```python
from build123d import *

# Parameters (mm, degrees)
SKETCH_1_R          = 1.45
EXTRUDE_1_DEPTH     = 3
SKETCH_3_R          = 1.95
CUT_EXTRUDE_2_DEPTH = 77.216796049
FILLET_1_R          = 5
SKETCH_4_R          = 10
CUT_EXTRUDE_3_DEPTH = 77.216796049
SKETCH_5_R          = 2.213245743
CUT_EXTRUDE_4_DEPTH = 77.216796049
FILLET_2_R          = 10
FILLET_3_R          = 3
FILLET_4_R          = 8


with BuildPart() as part:
    # 草图1 → 凸台-拉伸1 (new body)
    with BuildSketch(Plane.XY):
        with BuildLine():
            Line((-30, 31), (30, 31))
            Line((30, 31), (30, -40))
            ThreePointArc((30, -40), (0, -70), (-30, -40))
            Line((-30, -40), (-30, 31))
        make_face()
        with Locations((-20, 26)):
            Circle(SKETCH_1_R, mode=Mode.SUBTRACT)
        with Locations((-20, 16)):
            Circle(SKETCH_1_R, mode=Mode.SUBTRACT)
        with Locations((-20, 6)):
            Circle(SKETCH_1_R, mode=Mode.SUBTRACT)
        with Locations((-8, 26)):
            Circle(SKETCH_1_R, mode=Mode.SUBTRACT)
        with Locations((-8, 16)):
            Circle(SKETCH_1_R, mode=Mode.SUBTRACT)
        with Locations((-8, 6)):
            Circle(SKETCH_1_R, mode=Mode.SUBTRACT)
        with Locations(Location((8, 6, 0), (0, 0, 180))):
            Circle(SKETCH_1_R, mode=Mode.SUBTRACT)
        with Locations(Location((8, 16, 0), (0, 0, 180))):
            Circle(SKETCH_1_R, mode=Mode.SUBTRACT)
        with Locations(Location((8, 26, 0), (0, 0, 180))):
            Circle(SKETCH_1_R, mode=Mode.SUBTRACT)
        with Locations(Location((20, 6, 0), (0, 0, 180))):
            Circle(SKETCH_1_R, mode=Mode.SUBTRACT)
        with Locations(Location((20, 16, 0), (0, 0, 180))):
            Circle(SKETCH_1_R, mode=Mode.SUBTRACT)
        with Locations(Location((20, 26, 0), (0, 0, 180))):
            Circle(SKETCH_1_R, mode=Mode.SUBTRACT)
    extrude(amount=EXTRUDE_1_DEPTH)

    # 草图3 → 切除-拉伸2 (cut, through all)
    with BuildSketch(Plane.XY.offset(3)):
        with Locations((-21.75, -40)):
            Circle(SKETCH_3_R)
        with Locations((-13.980630511, -23.338533362)):
            Circle(SKETCH_3_R)
        with Locations((-13.980630511, -56.661466638)):
            Circle(SKETCH_3_R)
        with Locations((21.75, -40)):
            Circle(SKETCH_3_R)
        with Locations((13.980630511, -23.338533362)):
            Circle(SKETCH_3_R)
        with Locations((13.980630511, -56.661466638)):
            Circle(SKETCH_3_R)
    extrude(amount=-CUT_EXTRUDE_2_DEPTH, mode=Mode.SUBTRACT)

    # 圆角1
    fillet_1_edges = [part.edges().sort_by_distance(p)[0] for p in [
        (-30, 31, 1.5),
        (30, 31, 1.5),
    ]]
    fillet(fillet_1_edges, radius=FILLET_1_R)

    # 草图4 → 切除-拉伸3 (cut, through all)
    with BuildSketch(Plane.XY.offset(3)):
        with Locations((0, -40)):
            Circle(SKETCH_4_R)
    extrude(amount=-CUT_EXTRUDE_3_DEPTH, mode=Mode.SUBTRACT)

    # 草图5 → 切除-拉伸4 (cut, through all)
    with BuildSketch(Plane.XY.offset(3)):
        with Locations((-10.587343504, -27.656694111)):
            Circle(SKETCH_5_R)
        with Locations(Location((10.587343504, -27.656694111, 0), (0, 0, 180))):
            Circle(SKETCH_5_R)
        with BuildLine():
            Line((0, -22.555255147), (-8.212014753, -20.218285546))
            Line((-8.212014753, -20.218285546), (-10.389846713, -2.597786896))
            ThreePointArc((-10.389846713, -2.597786896), (-11.055900559, -0.155034313), (-12.38499612, 2))
            Line((-12.38499612, 2), (12.38499612, 2))
            ThreePointArc((12.38499612, 2), (11.055900559, -0.155034313), (10.389846713, -2.597786896))
            Line((10.389846713, -2.597786896), (8.212014753, -20.218285546))
            Line((8.212014753, -20.218285546), (0, -22.555255147))
        make_face()
        with BuildLine():
            ThreePointArc((-23.179978152, -59.044385338), (0, -64.997150083), (23.179978152, -59.044385338))
            ThreePointArc((23.179978152, -59.044385338), (0, -70), (-23.179978152, -59.044385338))
        make_face()
    extrude(amount=-CUT_EXTRUDE_4_DEPTH, mode=Mode.SUBTRACT)

    # 圆角2
    fillet_2_edges = [part.edges().sort_by_distance(p)[0] for p in [
        (23.179978152, -59.044385338, 1.5),
        (-23.179978152, -59.044385338, 1.5),
    ]]
    fillet(fillet_2_edges, radius=FILLET_2_R)

    # 圆角3
    fillet_3_edges = [part.edges().sort_by_distance(p)[0] for p in [
        (8.212014753, -20.218285546, 1.5),
        (-8.212014753, -20.218285546, 1.5),
        (-12.38499612, 2, 1.5),
        (12.38499612, 2, 1.5),
    ]]
    fillet(fillet_3_edges, radius=FILLET_3_R)

    # 圆角4
    fillet_4_edges = [part.edges().sort_by_distance(p)[0] for p in [
        (0, -22.555255147, 1.5),
    ]]
    fillet(fillet_4_edges, radius=FILLET_4_R)


solid = part.part
```
The listing builds one solid part. Answer for the finished solid, in the listing's coordinates (mm). A direction names the side the tool comes from. Round coordinates to 2 decimals unless told otherwise and drop trailing zeros. Loops run counter-clockwise (first coordinate to the right, second up) from the corner with the lowest first, then second, coordinate; pieces in that order, holes last. Notation, with made-up numbers: (88, 17) - (113, 17) arc R20 cw to (113, 42) - close; hole circle Ø5 at (20, 34.25). An arc over 180 degrees is marked (long way). Return JSON: item names as keys, results as strings. Group by question number.
1. Consider probe 1 along Y at (x, z) = (0, 1.8); probe 2 along Y at (x, z) = (-14, 1.95) (3 decimals); probe 3 along Y at (x, z) = (-20, 0.8). Determine where each line is inside the solid, lowest interval first.
2. The part is cut by section A-A on x = 0. Determine the outline of the cut face in (y, z).
3. The part is cut by section B-B on y = 16. Determine the outline of the cut face in (x, z), then the cut area to 3 significant figures.
4. The part is cut by section C-C on y = -44. Determine the outline of the cut face in (x, z).
5. The part is cut by section D-D on y = -26.5. Determine the outline of the cut face in (x, z).
6. Which of the six approach directions +Z, -Z, +X, -X, +Y, -Y give full straight-line access (tool end or side, diameter ignored) to faces 1 (the flat face through (30, -7, 1)), 2 (the cylindrical face through (-0.031, -22.238, 1.479))?
Resolved:
{
 "1": {"probe 1": "y = -65 to -50, -30 to -22.24, 2 to 31", "probe 2": "y = -62.915 to -58.611, -54.712 to -25.288, -21.389 to 31", "probe 3": "y = -60.64 to -40.86, -39.14 to 4.55, 7.45 to 14.55, 17.45 to 24.55, 27.45 to 31"},
 "2": {"outline": "(-65, 0) - (-50, 0) - (-50, 3) - (-65, 3) - close; (-30, 0) - (-22.24, 0) - (-22.24, 3) - (-30, 3) - close; (2, 0) - (31, 0) - (31, 3) - (2, 3) - close"},
 "3": {"outline": "(-30, 0) - (-21.45, 0) - (-21.45, 3) - (-30, 3) - close; (-18.55, 0) - (-9.45, 0) - (-9.45, 3) - (-18.55, 3) - close; (-6.55, 0) - (6.55, 0) - (6.55, 3) - (-6.55, 3) - close; (9.45, 0) - (18.55, 0) - (18.55, 3) - (9.45, 3) - close; (21.45, 0) - (30, 0) - (30, 3) - (21.45, 3) - close", "area": "145 mm²"},
 "4": {"outline": "(-29.73, 0) - (-9.17, 0) - (-9.17, 3) - (-29.73, 3) - close; (9.17, 0) - (29.73, 0) - (29.73, 3) - (9.17, 3) - close"},
 "5": {"outline": "(-30, 0) - (-12.47, 0) - (-12.47, 3) - (-30, 3) - close; (-8.7, 0) - (8.7, 0) - (8.7, 3) - (-8.7, 3) - close; (12.47, 0) - (30, 0) - (30, 3) - (12.47, 3) - close"},
 "6": {"face 1": "+Z, -Z, +X, +Y, -Y", "face 2": "+Z, -Z"}
}
